The model under review builds one solid part; all positions refer to its coordinate system, in mm. A direction names the side the tool comes from. Give positions to 0.01 mm unless a question says otherwise; leave off trailing zeros. Order: outer loops, then holes, each group sorted by start corner. A loop starts at its lowest first (then second) coordinate and runs counter-clockwise, first axis right, second up. Notation, with made-up numbers: (-2.5, -16) -> (28.5, -16) arc R25 cw to (28.5, 11) -> close; hole circle Ø5 at (1.25, -9). An arc over 180 degrees is marked (long way). Answer as a JSON object with one key per item and string values. Group by question number.
from build123d import *

# Parameters (mm, degrees)
EXTRUDE_THIN1_DEPTH = 206.375
FILLET1_R           = 1.016


with BuildPart() as part:
    # Sketch1 → Extrude-Thin1 (new body)
    with BuildSketch(Plane.XY):
        with BuildLine():
            Line((-1.01402142, 20.6375), (-1.41089642, 14.2875))
            Line((-1.41089642, 14.2875), (-12.7, 14.2875))
            Line((-12.7, 14.2875), (-12.7, 11.1125))
            ThreePointArc((-12.7, 11.1125), (-10.421749313, 10.393450043), (-8.969036168, 8.496852156))
            Line((-8.969036168, 8.496852156), (-7.699713832, 4.996897844))
            ThreePointArc((-7.699713832, 4.996897844), (-6.247000687, 3.100299957), (-3.96875, 2.38125))
            Line((-3.96875, 2.38125), (-3.96875, 0))
            Line((-3.96875, 0), (0, 0))
            Line((0, 0), (-0.396875, 3.150097655))
            Line((-0.396875, 3.150097655), (-1.40490625, 3.023097655))
            Line((-1.40490625, 3.023097655), (-1.152035714, 1.016))
            Line((-1.152035714, 1.016), (-2.95275, 1.016))
            Line((-2.95275, 1.016), (-2.95275, 3.57755044))
            ThreePointArc((-2.95275, 3.57755044), (-5.215232033, 3.673245416), (-6.744587091, 5.343291996))
            Line((-6.744587091, 5.343291996), (-8.013909427, 8.843246308))
            ThreePointArc((-8.013909427, 8.843246308), (-9.435411883, 10.910737787), (-11.684, 12.023860302))
            Line((-11.684, 12.023860302), (-11.684, 13.2715))
            Line((-11.684, 13.2715), (-0.456413979, 13.2715))
            Line((-0.456413979, 13.2715), (0, 20.574123661))
            Line((0, 20.574123661), (-1.01402142, 20.6375))
        make_face()
    extrude(amount=-EXTRUDE_THIN1_DEPTH)

    # Fillet1
    fillet1_edges = [part.edges().sort_by_distance(p)[0] for p in [
        (-3.96875, 0, -103.1875),
        (-12.7, 11.1125, -103.1875),
        (-12.7, 14.2875, -103.1875),
        (-0.456413979, 13.2715, -103.1875),
        (-2.95275, 3.57755044, -103.1875),
    ]]
    fillet(fillet1_edges, radius=FILLET1_R)


solid = part.part
1. Take a section at A-A on z = -130. Give the boundary of the cut face in (x, y), plus the area to 3 significant figures.
2. For probe 1 along Y at (x, z) = (-4, -165.5); probe 2 along Y at (x, z) = (-2, -112); probe 3 along X at (y, z) = (2, -22), list the stretches that pass through material, from the lowest coordinate up. Write a range as [from, to].
3. Take a section at B-B on y = 18.75. Give the boundary of the cut face in (x, z) (3 decimals), plus the area to 3 significant figures.
4. Machinability: for faces 4 (the flat face through (-7.37, 7.07, -101.74)), 5 (the flat face through (-8.3, 8.8, 0)), which of the approach directions +Z, -Z, +X, -X, +Y, -Y give a long, thin tool a straight path to every point of the face, cutting with its end or side? Answer none if there is none.
5. Draft analysis for pull direction Y (two halves, no side actions). For faces 1 (the flat face through (-6, 14.288, -102)), 2 (the cylindrical face through (-6.275, 3.12, -101.743)), 3 (the cylindrical face through (-9.41, 10.89, -101.74)), state which applies: pulls with the +Y half, pulls with the -Y half, needs draft (parallel to the pull), parting line crosses it, or undercut.
6. For pin 1 (1.5 mm diameter, centred on x = -7.5, z = -121.5, fed in from +Y); pin 2 (1 mm diameter, centred on y = 6, z = -83, fed in from -X); pin 3 (0.7 mm diameter, centred on y = 2, z = -55.5, fed in from +X), all flat-tipped, find the tip position at first contact; note any pin that passes through.
Checks:
{
 "1": {"outline": "(-12.7, 12.02) arc R1.02 ccw to (-11.89, 11.03) arc R3.97 cw to (-8.97, 8.5) -> (-7.7, 5) arc R3.97 ccw to (-3.97, 2.38) -> (-3.97, 1.02) arc R1.02 ccw to (-2.95, 0) -> (0, 0) -> (-0.4, 3.15) -> (-1.4, 3.02) -> (-1.15, 1.02) -> (-2.95, 1.02) -> (-2.95, 2.38) arc R1.02 ccw to (-3.97, 3.4) arc R2.95 cw to (-6.74, 5.34) -> (-8.01, 8.84) arc R4.98 ccw to (-11.68, 12.02) -> (-11.68, 13.27) -> (-1.41, 13.27) arc R1.02 ccw to (-0.4, 14.22) -> (0, 20.57) -> (-1.01, 20.64) -> (-1.41, 14.29) -> (-11.68, 14.29) arc R1.02 ccw to (-12.7, 13.27) -> close", "area": "41.2 mm2"},
 "2": {"probe 1": "y = [2.38, 3.4], [13.27, 14.29]", "probe 2": "y = [0, 1.02], [13.27, 14.29]", "probe 3": "x = [-3.97, -2.95], [-1.28, -0.25]"},
 "3": {"outline": "(-1.132, -206.375) -> (-0.114, -206.375) -> (-0.114, 0) -> (-1.132, 0) -> close", "area": "210 mm2"},
 "4": {"face 4": "+Z, -Z, +X", "face 5": "+Z, +X, -X, +Y, -Y"},
 "5": {"face 1": "pulls with the +Y half", "face 2": "pulls with the -Y half", "face 3": "undercut"},
 "6": {"pin 1": "stops at y = 14.29", "pin 2": "stops at x = -8.24", "pin 3": "stops at x = -0.21"}
}
